from build123d import *

# Parameters (mm, degrees)
F9_T = -2.5


with BuildPart() as f4:
    # F0 (on Top) → F4 section 0
    with BuildSketch(Plane.XY):
        Polygon((27.2798002192, 15.75), (0, 31.5), (-27.2798002192, 15.75), (-27.2798002192, -15.75), (0, -31.5), (27.2798002192, -15.75), align=None)
    # F2 (on offset) → F4 section 1
    with BuildSketch(Plane.XY.offset(20)):
        Polygon((-38.9711431703, -22.5), (0, -45), (38.9711431703, -22.5), (38.9711431703, 22.5), (0, 45), (-38.9711431703, 22.5), align=None)
    loft()


with BuildPart() as f5_1:
    # F5: copy of F4
    add(f4.part.moved(Location((0, 133, 0))))


with BuildPart() as f4_1:
    add(f4.part)

    # F4_face (on face) → F8 section 0
    with BuildSketch(Plane.XY.offset(20)):
        Polygon((38.9711431703, 22.5), (0, 45), (-38.9711431703, 22.5), (-38.9711431703, -22.5), (0, -45), (38.9711431703, -22.5), align=None)
    # F6 (on offset) → F8 section 1
    with BuildSketch(Plane.XY.offset(60)):
        Polygon((-38.9711431703, -22.5), (0, -45), (38.9711431703, -22.5), (38.9711431703, 22.5), (0, 45), (-38.9711431703, 22.5), align=None)
    loft()

    # F9
    f9_openings = [f4_1.faces().sort_by_distance(p)[0] for p in [
        (0, 0, 60),
    ]]
    offset(amount=F9_T, openings=f9_openings, kind=Kind.INTERSECTION)


solid = f4_1.part
Verification items for the finished model (mm, model axes). A direction names the side the tool comes from. Coordinates: 2 decimals unless noted, no trailing zeros. Write each loop counter-clockwise with the first axis right and the second up, starting at its lowest first coordinate (ties: lowest second). Pieces come first, ordered by that corner, then holes. Notation, with made-up numbers: M 67.25,20 L 99.25,20 A11 ccw 99.25,31 Z; hole C 12.25,-17.5 d1. An arc over 180 degrees is marked long. Use a Markdown table: item, result.
Q1. Draft check along X on faces 1 (the face through (38.971, 0, 40)), 2 (the face through (17.98, -31.732, 40.614)), 3 (the face through (-36.471, 0, 41)), 4 (the face through (-19.21, 33.91, 40.28)). Enter one of: +X half, -X half, draft (parallel to the pull), parting line (faces both ways), or undercut.
Reply:
| item | result |
|---|---|
| face 1 | +X half |
| face 2 | undercut |
| face 3 | undercut |
| face 4 | -X half |
Q2. Go/stop test with flat-tipped pins: P1, Ø1, axis at y = 10, z = 16, coming from the +X side; P2, Ø3, axis at x = -12, z = 29.5, coming from the -Y side; P3, Ø2, axis at y = -1, z = 14, coming from the -X side. Record where each tip stops, or that it passes through.
Reply:
| item | result |
|---|---|
| P1 | stops at x = 36.93 |
| P2 | stops at y = -38.94 |
| P3 | stops at x = -36.05 |
Q3. Sectioned sample at A-A, the plane z = 29. Record the boundary of the cut face in (x, y).
Reply:
| item | result |
|---|---|
| outline | M -38.97,-22.5 L 0,-45 L 38.97,-22.5 L 38.97,22.5 L 0,45 L -38.97,22.5 Z; hole M -36.47,-21.06 L 0,-42.11 L 36.47,-21.06 L 36.47,21.06 L 0,42.11 L -36.47,21.06 Z |
Q4. Thickness scan on line 1 (X direction, y = 7, z = 33.5); line 2 (Z direction, x = 15, y = -19.5); line 3 (Y direction, x = 30, z = 34). Record the ranges inside material, lowest first.
Reply:
| item | result |
|---|---|
| line 1 | x = -38.97 to -36.47, 36.47 to 38.97 |
| line 2 | z = 0 to 2.5 |
| line 3 | y = -27.68 to -24.79, 24.79 to 27.68 |
Q5. Set-up check for faces 5 (the face through (18.49, 31.44, 40.61)), 6 (the face through (-38.971, 0, 40)): record each of +Z, -Z, +X, -X, +Y, -Y from which the full face is reachable in a straight line by a thin tool's end or side.
Reply:
| item | result |
|---|---|
| face 5 | +Z |
| face 6 | +Z, -Z, -X, +Y, -Y |
